CAD build for the part. Positions are in the model's coordinates, mm. Give positions to 0.01 mm unless a question says otherwise; leave off trailing zeros. One line per question, with ' | ' between items. Start each with the question number.
1. Wall check: L1, parallel to Z at x = 10.16, y = 3.1; L2, parallel to X at y = 0.85, z = 0; L3, parallel to X at y = 2.95, z = -63. Give the ranges that are in metal, low to high.
2. Cut at A-A, the plane y = 1.1. Count the separate pieces of the cut face and the enclosed holes in it, then the cut area to 3 significant figures.
3. Flat gauge pins, fed straight in: pin 1 (1 mm diameter, centred on y = 3, z = -50.5, fed in from +X); pin 2 (1.3 mm diameter, centred on x = 110.45, z = -4.78, fed in from +Y). Where does each tip first touch, or does it go through?
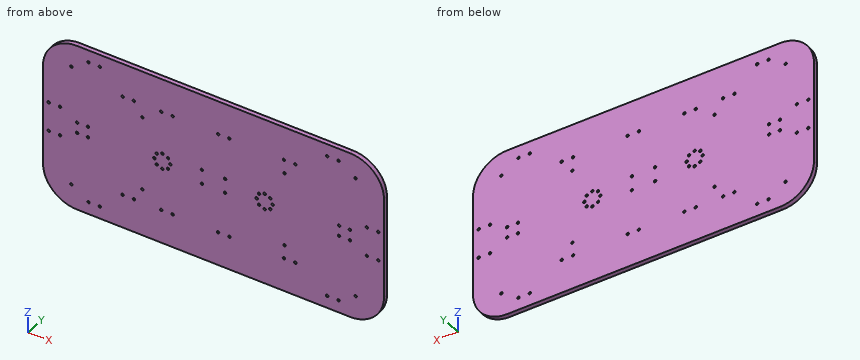
```python
from build123d import *

# Parameters (mm, degrees)
SKETCH_1_W                            = 300
SKETCH_1_H                            = 150
EXTRUDE_1_DEPTH                       = 4
FILLET_4_R                            = 30
FILLET_5_R                            = 30
FILLET_6_R                            = 30
FILLET_7_R                            = 30
HOLE_WIZARD_2_2_2_2_1_D               = 2.2
PATTERN_CIRCULAR_1_COUNT              = 8
MIRROR_1_COPY_1_D                     = 2.2
MIRROR_1_COPY_2_D                     = 2.2
MIRROR_1_COPY_3_D                     = 2.2
MIRROR_1_COPY_4_D                     = 2.2
MIRROR_1_COPY_5_D                     = 2.2
MIRROR_1_COPY_6_D                     = 2.2
MIRROR_1_COPY_7_D                     = 2.2
HOLE_WIZARD_2_2_2_2_2_D               = 2.2
HOLE_WIZARD_2_2_2_2_4_D               = 2.2
F_2_2_2_2_DIAMETER_HOLE1_D            = 2.2
MIRROR_5_AT_THE_SECOND_PLANE_COPY_1_D = 2.2
HOLE_WIZARD_2_2_2_2_6_D               = 2.2
F_2_2_2_2_DIAMETER_HOLE2_D            = 2.2
MIRROR_6_AT_THE_SECOND_PLANE_COPY_1_D = 2.2
F_2_2_2_2_DIAMETER_HOLE3_D            = 2.2
F_2_2_2_2_DIAMETER_HOLE4_D            = 2.2
MIRROR_8_AT_THE_SECOND_PLANE_COPY_1_D = 2.2


with BuildPart() as part:
    # 草图1 → 凸台-拉伸1 (new body)
    with BuildSketch(Plane(origin=(0, 0, 0), x_dir=(1, 0, 0), z_dir=(0, 1, 0))):
        Rectangle(SKETCH_1_W, SKETCH_1_H)
    extrude(amount=EXTRUDE_1_DEPTH)

    # 圆角4
    fillet_4_edges = [part.edges().sort_by_distance(p)[0] for p in [
        (-150, 2, 75),
    ]]
    fillet(fillet_4_edges, radius=FILLET_4_R)

    # 圆角5
    fillet_5_edges = [part.edges().sort_by_distance(p)[0] for p in [
        (-150, 2, -75),
    ]]
    fillet(fillet_5_edges, radius=FILLET_5_R)

    # 圆角6
    fillet_6_edges = [part.edges().sort_by_distance(p)[0] for p in [
        (150, 2, -75),
    ]]
    fillet(fillet_6_edges, radius=FILLET_6_R)

    # 圆角7
    fillet_7_edges = [part.edges().sort_by_distance(p)[0] for p in [
        (150, 2, 75),
    ]]
    fillet(fillet_7_edges, radius=FILLET_7_R)

    # Ø2.2 (2.2) 直径孔1 (through all)
    with Locations(Plane(origin=(0, 0, 0), x_dir=(-1, 0, 0), z_dir=(0, -1, 0))):
        with Locations((45, -7.02)):
            hole_wizard_2_2_2_2_1 = Hole(HOLE_WIZARD_2_2_2_2_1_D / 2)

    # 阵列(圆周)1: Ø2.2 (2.2) 直径孔1 ×8 about axis
    pattern_circular_1_axis = Axis((-45, 0, 0), (0, 1, 0))
    for i in range(1, PATTERN_CIRCULAR_1_COUNT):
        add(hole_wizard_2_2_2_2_1.rotate(pattern_circular_1_axis, i * 360 / PATTERN_CIRCULAR_1_COUNT), mode=Mode.SUBTRACT)

    # 镜向1: Ø2.2 (2.2) 直径孔1 across plane
    add(hole_wizard_2_2_2_2_1.mirror(Plane(origin=(0, 0, 0), x_dir=(0, 0, 1), z_dir=(1, 0, 0))), mode=Mode.SUBTRACT)

    # 镜向1 copy 1 (through all)
    with Locations(Plane(origin=(13.180194847, 0, -31.819805153), x_dir=(0.7071067811865476, 0, 0.7071067811865475), z_dir=(0, -1, 0))):
        with Locations((45, 7.02)):
            Hole(MIRROR_1_COPY_1_D / 2)

    # 镜向1 copy 2 (through all)
    with Locations(Plane(origin=(45, 0, -45), x_dir=(0, 0, 1), z_dir=(0, -1, 0))):
        with Locations((45, 7.02)):
            Hole(MIRROR_1_COPY_2_D / 2)

    # 镜向1 copy 3 (through all)
    with Locations(Plane(origin=(76.819805153, 0, -31.819805153), x_dir=(-0.7071067811865475, 0, 0.7071067811865476), z_dir=(0, -1, 0))):
        with Locations((45, 7.02)):
            Hole(MIRROR_1_COPY_3_D / 2)

    # 镜向1 copy 4 (through all)
    with Locations(Plane(origin=(90, 0, 0), x_dir=(-1, 0, 0), z_dir=(0, -1, 0))):
        with Locations((45, 7.02)):
            Hole(MIRROR_1_COPY_4_D / 2)

    # 镜向1 copy 5 (through all)
    with Locations(Plane(origin=(76.819805153, 0, 31.819805153), x_dir=(-0.7071067811865477, 0, -0.7071067811865475), z_dir=(0, -1, 0))):
        with Locations((45, 7.02)):
            Hole(MIRROR_1_COPY_5_D / 2)

    # 镜向1 copy 6 (through all)
    with Locations(Plane(origin=(45, 0, 45), x_dir=(0, 0, -1), z_dir=(0, -1, 0))):
        with Locations((45, 7.02)):
            Hole(MIRROR_1_COPY_6_D / 2)

    # 镜向1 copy 7 (through all)
    with Locations(Plane(origin=(13.180194847, 0, 31.819805153), x_dir=(0.7071067811865474, 0, -0.7071067811865477), z_dir=(0, -1, 0))):
        with Locations((45, 7.02)):
            Hole(MIRROR_1_COPY_7_D / 2)

    # Ø2.2 (2.2) 直径孔2 (through all)
    with Locations(Plane(origin=(0, 0, 0), x_dir=(-1, 0, 0), z_dir=(0, -1, 0))):
        with Locations((120, 4.78), (120, -4.775), (110.45, -4.775), (110.45, 4.78)):
            hole_wizard_2_2_2_2_2 = Hole(HOLE_WIZARD_2_2_2_2_2_D / 2)

    # 镜向2: Ø2.2 (2.2) 直径孔2 across plane
    add(hole_wizard_2_2_2_2_2.mirror(Plane(origin=(0, 0, 0), x_dir=(0, 0, 1), z_dir=(1, 0, 0))), mode=Mode.SUBTRACT)

    # Ø2.2 (2.2) 直径孔4 (through all)
    with Locations(Plane(origin=(0, 4, 0), x_dir=(1, 0, 0), z_dir=(0, 1, 0))):
        with Locations((100, -64), (110, -64), (-100, -64), (-110, -64)):
            hole_wizard_2_2_2_2_4 = Hole(HOLE_WIZARD_2_2_2_2_4_D / 2)

    # 镜向4: Ø2.2 (2.2) 直径孔4 across plane
    add(hole_wizard_2_2_2_2_4.mirror(Plane.XY), mode=Mode.SUBTRACT)

    # Ø2.2 (2.2) Diameter Hole1 (through all)
    with Locations(Plane(origin=(0, 4, 0), x_dir=(1, 0, 0), z_dir=(0, 1, 0))):
        with Locations((-125, 54)):
            f_2_2_2_2_diameter_hole1 = Hole(F_2_2_2_2_DIAMETER_HOLE1_D / 2)

    # 镜向5: Ø2.2 (2.2) Diameter Hole1 across plane
    add(f_2_2_2_2_diameter_hole1.mirror(Plane(origin=(0, 0, 0), x_dir=(0, 0, 1), z_dir=(1, 0, 0))), mode=Mode.SUBTRACT)

    # 镜向5 at the second plane: Ø2.2 (2.2) Diameter Hole1 across plane
    add(f_2_2_2_2_diameter_hole1.mirror(Plane.XY), mode=Mode.SUBTRACT)

    # 镜向5 at the second plane copy 1 (through all)
    with Locations(Plane(origin=(0, 4, 0), x_dir=(-1, 0, 0), z_dir=(0, 1, 0))):
        with Locations((-125, 54)):
            Hole(MIRROR_5_AT_THE_SECOND_PLANE_COPY_1_D / 2)

    # Ø2.2 (2.2) 直径孔6 (through all)
    with Locations(Plane(origin=(0, 4, 0), x_dir=(1, 0, 0), z_dir=(0, 1, 0))):
        with Locations((-62.5, 33), (-62.5, -33), (62.5, -33), (62.5, 33)):
            Hole(HOLE_WIZARD_2_2_2_2_6_D / 2)

    # Ø2.2 (2.2) Diameter Hole2 (through all)
    with Locations(Plane(origin=(0, 4, 0), x_dir=(1, 0, 0), z_dir=(0, 1, 0))):
        with Locations((-145, 13), (-135, 13)):
            f_2_2_2_2_diameter_hole2 = Hole(F_2_2_2_2_DIAMETER_HOLE2_D / 2)

    # 镜向6: Ø2.2 (2.2) Diameter Hole2 across plane
    add(f_2_2_2_2_diameter_hole2.mirror(Plane(origin=(0, 0, 0), x_dir=(0, 0, 1), z_dir=(1, 0, 0))), mode=Mode.SUBTRACT)

    # 镜向6 at the second plane: Ø2.2 (2.2) Diameter Hole2 across plane
    add(f_2_2_2_2_diameter_hole2.mirror(Plane.XY), mode=Mode.SUBTRACT)

    # 镜向6 at the second plane copy 1 (through all)
    with Locations(Plane(origin=(0, 4, 0), x_dir=(-1, 0, 0), z_dir=(0, 1, 0))):
        with Locations((-145, 13), (-135, 13)):
            Hole(MIRROR_6_AT_THE_SECOND_PLANE_COPY_1_D / 2)

    # Ø2.2 (2.2) Diameter Hole3 (through all)
    with Locations(Plane(origin=(0, 4, 0), x_dir=(1, 0, 0), z_dir=(0, 1, 0))):
        with Locations((-80, 45), (-70, 45), (-46, 45), (-36, 45), (4, 45), (14, 45), (62, 45), (72, 45)):
            f_2_2_2_2_diameter_hole3 = Hole(F_2_2_2_2_DIAMETER_HOLE3_D / 2)

    # 镜向7: Ø2.2 (2.2) Diameter Hole3 across plane
    add(f_2_2_2_2_diameter_hole3.mirror(Plane.XY), mode=Mode.SUBTRACT)

    # Ø2.2 (2.2) Diameter Hole4 (through all)
    with Locations(Plane.XZ):
        with Locations((-10.16, 6.35)):
            f_2_2_2_2_diameter_hole4 = Hole(F_2_2_2_2_DIAMETER_HOLE4_D / 2)

    # 镜向8: Ø2.2 (2.2) Diameter Hole4 across plane
    add(f_2_2_2_2_diameter_hole4.mirror(Plane.XY), mode=Mode.SUBTRACT)

    # 镜向8 at the second plane: Ø2.2 (2.2) Diameter Hole4 across plane
    add(f_2_2_2_2_diameter_hole4.mirror(Plane(origin=(0, 0, 0), x_dir=(0, 0, 1), z_dir=(1, 0, 0))), mode=Mode.SUBTRACT)

    # 镜向8 at the second plane copy 1 (through all)
    with Locations(Plane(origin=(0, 0, 0), x_dir=(-1, 0, 0), z_dir=(0, -1, 0))):
        with Locations((-10.16, 6.35)):
            Hole(MIRROR_8_AT_THE_SECOND_PLANE_COPY_1_D / 2)


solid = part.part
```
Here are the results:
1) L1: -75 to -7.45, -5.25 to 5.25, 7.45 to 75 | L2: -150 to -53.12, -50.92 to -39.08, -36.88 to 36.88, 39.08 to 50.92, 53.12 to 150 | L3: -144 to -110.46, -109.54 to -100.46, -99.54 to 99.54, 100.46 to 109.54, 110.46 to 144
2) separate pieces: 1 | enclosed holes: 68 | area: 44,000 mm^2
3) pin 1: x = 149.58 | pin 2: through
